Autodesk Fusion 360 part; units mm, degrees
sketch "Sketch1" plane through (0, 0, 0) normal (0, 0, 1) x (1, 0, 0)
  line L0 (10, 0) -> (182, 0)
  line L1 (192, 10) -> (192, 133.562)
  line L2 (182, 143.562) -> (10, 143.562)
  line L3 (0, 133.562) -> (0, 10)
  line L4 (126.5, 133.062) -> (126.5, 10.5)
  circle A0 centre (126.5, 133.062) radius 3.5
  circle A1 centre (126.5, 10.5) radius 3.5
  line L5 (126.5, 71.781) -> (192, 71.781)
  line L6 (177, 71.781) -> (76, 71.781)
  line L7 (76, 82.781) -> (76, 60.781)
  circle A2 centre (76, 82.781) radius 3.5
  circle A3 centre (76, 60.781) radius 3.5
  line L8 (177, 82.781) -> (177, 60.781)
  circle A4 centre (177, 82.781) radius 3.5
  circle A5 centre (177, 60.781) radius 3.5
  line L9 (11, 106.781) -> (61, 106.781)
  line L10 (61, 106.781) -> (61, 36.781)
  line L11 (61, 36.781) -> (11, 36.781)
  line L12 (11, 36.781) -> (11, 106.781)
  line L13 (11, 71.781) -> (0, 71.781)
  circle A6 centre (61, 106.781) radius 1.55
  circle A7 centre (11, 106.781) radius 1.55
  circle A8 centre (11, 36.781) radius 1.55
  circle A9 centre (61, 36.781) radius 1.55
  arc A10 (10, 143.562) -> (0, 133.562) centre (10, 133.562) ccw
  arc A11 (192, 133.562) -> (182, 143.562) centre (182, 133.562) ccw
  arc A12 (182, 0) -> (192, 10) centre (182, 10) ccw
  arc A13 (0, 10) -> (10, 0) centre (10, 10) ccw
  point P0 (192, 0)
  point P1 (192, 143.562)
  point P2 (76, 71.781)
  point P3 (126.5, 71.781)
  dimension "d1" = 143.562
  dimension "d3" = 7
  dimension "d4" = 7
  dimension "d5" = 122.562
  dimension "d6" = 90
  dimension "d7" = 101
  dimension "d8" = 22
  dimension "d9" = 7
  dimension "d10" = 7
  dimension "d11" = 15
  dimension "d12" = 50
  dimension "d13" = 70
  dimension "d14" = 15
  dimension "d15" = 90
  dimension "d16" = 3.1
  dimension "d17" = 3.1
  dimension "d18" = 3.1
  dimension "d19" = 3.1
  dimension "d20" = 10
  dimension "d21" = 10
  dimension "d22" = 10
  dimension "d23" = 10
  dimension "d42" = 11
extrude "Extrude1" add sketch "Sketch1" along normal blind 10 contours L9 L10 L11 L12 A6 A7 A8 A9 | L0 L1 L2 L3 A10 A11 A12 A13
extrude "Extrude2" add 1 faces at (162.3446, 23.2161, 10) along direction (0, 0, 1) blind 1
extrude "Extrude3" add 1 faces at (162.3446, 23.2161, 0) along direction (0, 0, -1) blind 1
equation "d7 = 90 mm + 11 mm"
Build history of the part. All positions in model axes, mm. Round coordinates to 2 decimals unless told otherwise and drop trailing zeros. Loops run counter-clockwise (first coordinate to the right, second up) from the corner with the lowest first, then second, coordinate; pieces in that order, holes last. Notation, with made-up numbers: (39.25, -13.5) -> (70.25, -13.5) arc R10 cw to (70.25, 4.5) -> close; hole circle Ø10 at (9.5, 44). An arc over 180 degrees is marked (long way). Answer in a Markdown table with one row per item.
Item 1: Mould opens along X. For faces 1 (the cylindrical face through (180.34, 61.83, 5.08)), 2 (the cylindrical face through (3.007, 140.71, 5.084)), 3 (the flat face through (95, 0, 5)), 4 (the cylindrical face through (188.99, 2.85, 5.08)) say: +X half, -X half, draft (parallel to the pull), parting line (faces both ways), or undercut.
Answers below:
| item | result |
|---|---|
| face 1 | undercut |
| face 2 | -X half |
| face 3 | draft |
| face 4 | +X half |
Item 2: Saw through at A-A (x = 77.5). Write the cut outline in (y, z), and give its area (3 significant figures).
Answers below:
| item | result |
|---|---|
| outline | (0, -1) -> (57.62, -1) -> (57.62, 11) -> (0, 11) -> close; (63.94, -1) -> (79.62, -1) -> (79.62, 11) -> (63.94, 11) -> close; (85.94, -1) -> (143.56, -1) -> (143.56, 11) -> (85.94, 11) -> close |
| area | 1,570 mm² |
Item 3: Drill centre lines: L1, parallel to Y at x = 177, z = 8; L2, parallel to Y at x = 61, z = 4.5; L3, parallel to X at y = 86, z = 0. Where is each one in solid material? Low to high. Write a range as [from, to].
Answers below:
| item | result |
|---|---|
| L1 | y = [0, 57.28], [64.28, 79.28], [86.28, 143.56] |
| L2 | y = [0, 35.23], [38.33, 105.23], [108.33, 143.56] |
| L3 | x = [0, 74.63], [77.37, 175.63], [178.37, 192] |
Item 4: Saw through at B-B (x = 126.5). Write the cut outline in (y, z), and give its area (3 significant figures).
Answers below:
| item | result |
|---|---|
| outline | (0, -1) -> (7, -1) -> (7, 11) -> (0, 11) -> close; (14, -1) -> (129.56, -1) -> (129.56, 11) -> (14, 11) -> close; (136.56, -1) -> (143.56, -1) -> (143.56, 11) -> (136.56, 11) -> close |
| area | 1,550 mm² |
